Here's how the part is built. I have some questions about the finished solid (model axes, mm). A direction names the side the tool comes from. Coordinates: 2 decimals unless noted, no trailing zeros. Loops run counter-clockwise (first coordinate to the right, second up) from the corner with the lowest first, then second, coordinate; pieces in that order, holes last.
from build123d import *

# Parameters (mm, degrees)
BASE_DEPTH    = 3.2
SKETCH2_R     = 6.5
HOLES_DEPTH   = 120.412059692
CUTAWAY_DEPTH = 120.412059692


with BuildPart() as part:
    # Sketch1 → base (new body)
    with BuildSketch(Plane(origin=(0, 0, 0), x_dir=(1, 0, 0), z_dir=(0, 1, 0))):
        with BuildLine():
            ThreePointArc((4.25, 31.051933495), (-7.559468778, 28.546329643), (-8.351646544, 16.5))
            ThreePointArc((-8.351646544, 16.5), (-3.406586177, 0), (-8.351646544, -16.5))
            ThreePointArc((-8.351646544, -16.5), (-7.559468778, -28.546329643), (4.25, -31.051933495))
            ThreePointArc((4.25, -31.051933495), (8.5, -30.10386699), (12.75, -31.051933495))
            ThreePointArc((12.75, -31.051933495), (18.909452709, -31.816006843), (24.333333333, -28.798692685))
            ThreePointArc((24.333333333, -28.798692685), (61, -12.792156109), (97.666666667, -28.798692685))
            ThreePointArc((97.666666667, -28.798692685), (111.170389039, -29.869326471), (113.351646544, -16.5))
            ThreePointArc((113.351646544, -16.5), (108.406586177, 0), (113.351646544, 16.5))
            ThreePointArc((113.351646544, 16.5), (111.170389039, 29.869326471), (97.666666667, 28.798692685))
            ThreePointArc((97.666666667, 28.798692685), (61, 12.792156109), (24.333333333, 28.798692685))
            ThreePointArc((24.333333333, 28.798692685), (18.909452709, 31.816006843), (12.75, 31.051933495))
            ThreePointArc((12.75, 31.051933495), (8.5, 30.10386699), (4.25, 31.051933495))
        make_face()
    extrude(amount=-BASE_DEPTH)

    # Sketch2 → holes (cut, through all)
    with BuildSketch(Plane(origin=(0, 0, 0), x_dir=(1, 0, 0), z_dir=(0, 1, 0))):
        with Locations(Location((0, 22, 0), (0, 0, 270))):
            Circle(SKETCH2_R)
        with Locations(Location((17, 22, 0), (0, 0, 270))):
            Circle(SKETCH2_R)
        with Locations(Location((105, 22, 0), (0, 0, 270))):
            Circle(SKETCH2_R)
        with Locations(Location((105, -22, 0), (0, 0, 270))):
            Circle(SKETCH2_R)
        with Locations(Location((17, -22, 0), (0, 0, 270))):
            Circle(SKETCH2_R)
        with Locations(Location((0, -22, 0), (0, 0, 270))):
            Circle(SKETCH2_R)
    extrude(amount=-HOLES_DEPTH, mode=Mode.SUBTRACT)

    # Sketch3 → cutaway (cut, through all)
    with BuildSketch(Plane(origin=(0, 0, 0), x_dir=(-1, 0, 0), z_dir=(0, 1, 0))):
        with BuildLine():
            Line((-23.5, -6.500504863), (-23.5, 6.500504863))
            ThreePointArc((-23.5, 6.500504863), (-26, 10.830631882), (-31, 10.830631882))
            ThreePointArc((-31, 10.830631882), (-61.221365673, 2.792564466), (-91.38259727, 11.053410636))
            ThreePointArc((-91.38259727, 11.053410636), (-96.717445945, 10.882305495), (-98.858047687, 5.992754234))
            ThreePointArc((-98.858047687, 5.992754234), (-98.406586177, 0), (-98.858047687, -5.992754234))
            ThreePointArc((-98.858047687, -5.992754234), (-96.717445945, -10.882305495), (-91.38259727, -11.053410636))
            ThreePointArc((-91.38259727, -11.053410636), (-61.221365673, -2.792564466), (-31, -10.830631882))
            ThreePointArc((-31, -10.830631882), (-26, -10.830631882), (-23.5, -6.500504863))
        make_face()
    extrude(amount=-CUTAWAY_DEPTH, mode=Mode.SUBTRACT)


solid = part.part
Q1. Please list where these lines run through material, in increasing order: probe 1 along X at (y, z) = (-1.9, -22); probe 2 along X at (y, z) = (-0.7, 20); probe 3 along Z at (x, y) = (103, -1.75).
Q2. For faces 1 (the cylindrical face through (61.576, -1.578, -12.795)), 2 (the cylindrical face through (96.78, -1.58, -10.84)), which set-ups out of +Z, -Z, +X, -X, +Y, -Y let a thin tool reach every point of the face, with its end or its side?
Q3. Suppose I cut it at C-C on x = 105. Write out the boundary of the cut face in (y, z), and give its area (3 significant figures).
Q4. Suppose I cut it at D-D on y = -2.55. Write out the boundary of the cut face in (x, z), and give its area (3 significant figures).
Q5. We'd pull the mould along X, two halves only. Please class faces 3 (the cylindrical face through (108.408, -1.578, 0.245)), 4 (the cylindrical face through (-3.408, -1.578, -0.245)), 5 (the cylindrical face through (98.655, -1.578, -23.409)), 6 (the flat face through (52, -3.2, -8)): pulls with the +X half, pulls with the -X half, needs draft (parallel to the pull), parting line crosses it, or undercut.
Q6. Suppose I cut it at A-A on x = 90. Write out the boundary of the cut face in (y, z), and give its area (3 significant figures).
Q7. Suppose I cut it at B-B on z = -4.5. Write out the boundary of the cut face in (x, y), and give its area (3 significant figures).
Q8. Will these pins go through, and if not, where does the flat tip stop? P1, Ø11.5, axis at x = 0, z = 22, coming from the -Y side; P2, Ø1, axis at y = -2, z = 1, coming from the +X side.
Check values:
1. probe 1: x = -10 to -6.5, 6.5 to 10.5, 23.5 to 32.09, 89.91 to 98.5, 111.5 to 115
1. probe 2: x = -9.8 to -6.18, 6.18 to 10.82, 23.18 to 35.14, 86.86 to 98.82, 111.18 to 114.8
1. probe 3: z = -31.8 to -28.18, -15.82 to 15.82, 28.18 to 31.8
2. face 1: -Z, +Y, -Y
2. face 2: +Y, -Y
3. outline: (-3.2, -32) - (0, -32) - (0, -28.5) - (-3.2, -28.5) - close; (-3.2, -15.5) - (0, -15.5) - (0, 15.5) - (-3.2, 15.5) - close; (-3.2, 28.5) - (0, 28.5) - (0, 32) - (-3.2, 32) - close
3. area: 122 mm2
4. outline: (-8.35, -16.5) arc R10 ccw to (4.25, -31.05) arc R10 cw to (12.75, -31.05) arc R10 ccw to (24.33, -28.8) arc R50 cw to (97.67, -28.8) arc R10 ccw to (113.35, -16.5) arc R30 cw to (113.35, 16.5) arc R10 ccw to (97.67, 28.8) arc R50 cw to (24.33, 28.8) arc R10 ccw to (12.75, 31.05) arc R10 cw to (4.25, 31.05) arc R10 ccw to (-8.35, 16.5) arc R30 cw to start; hole circle Ø13 at (0, -22); hole circle Ø13 at (0, 22); hole circle Ø13 at (17, -22); hole circle Ø13 at (17, 22); hole (23.5, -6.5) arc R5 ccw to (31, -10.83) arc R60 cw to (91.38, -11.05) arc R5 ccw to (98.86, -5.99) arc R40 cw to (98.86, 5.99) arc R5 ccw to (91.38, 11.05) arc R60 cw to (31, 10.83) arc R5 ccw to (23.5, 6.5) - close; hole circle Ø13 at (105, -22); hole circle Ø13 at (105, 22)
4. area: 3,640 mm2
5. face 3: pulls with the +X half
5. face 4: pulls with the -X half
5. face 5: undercut
5. face 6: needs draft
6. outline: (-3.2, -22.06) - (0, -22.06) - (0, -10.27) - (-3.2, -10.27) - close; (-3.2, 10.27) - (0, 10.27) - (0, 22.06) - (-3.2, 22.06) - close
6. area: 75.5 mm2
7. outline: (-3.75, -3.2) - (23.5, -3.2) - (23.5, 0) - (-3.75, 0) - close; (46.79, -3.2) - (75.21, -3.2) - (75.21, 0) - (46.79, 0) - close; (98.66, -3.2) - (108.75, -3.2) - (108.75, 0) - (98.66, 0) - close
7. area: 210 mm2
8. P1: passes through
8. P2: stops at x = 108.44
